from build123d import *

# Parameters (mm, degrees)
BOSS_EXTRUDE1_DEPTH  = 160
SKETCH2_W            = 40
SKETCH2_H            = 2
CUT_EXTRUDE1_DEPTH   = 4
M4_CLEARANCE_HOLE1_D = 4.5
CUT_EXTRUDE2_REACH   = 163.357
SKETCH5_R            = 3.1


with BuildPart() as part:
    # Sketch1 → Boss-Extrude1 (new body)
    with BuildSketch(Plane.XY):
        Polygon((4, -4), (16, -4), (16, -10), (20, -10), (20, 0), (16, 0), (4, 0), align=None)
    extrude(amount=BOSS_EXTRUDE1_DEPTH)

    # Sketch2 → Cut-Extrude1 (cut)
    with BuildSketch(Plane(origin=(20, 0, 0), x_dir=(0, 0, -1), z_dir=(1, 0, 0))):
        with Locations((-140, -9)):
            Rectangle(SKETCH2_W, SKETCH2_H)
    extrude(amount=-CUT_EXTRUDE1_DEPTH, mode=Mode.SUBTRACT)

    # M4 Clearance Hole1 (through all)
    with Locations(Plane(origin=(0, -4, 0), x_dir=(-1, 0, 0), z_dir=(0, -1, 0))):
        with Locations((-10.128911503, -6.267286375), (-10.128911503, -23.38156703), (-10.128911503, -42.093180546), (-10.128911503, -63.314888558), (-9.444340277, -107.583827852), (-9.444340277, -150.244789298)):
            Hole(M4_CLEARANCE_HOLE1_D / 2)

    # Sketch5 → Cut-Extrude2 (cut, up to next)
    with BuildSketch(Plane.XZ.offset(4), mode=Mode.PRIVATE) as cut_extrude2_sk1:
        with Locations(Location((9, 138.897931951, 0), (0, 0, 270))):
            Circle(SKETCH5_R)
    cut_extrude2_tool1 = extrude(cut_extrude2_sk1.sketch, amount=-CUT_EXTRUDE2_REACH, mode=Mode.PRIVATE) & part.part
    add(cut_extrude2_tool1.solids().sort_by_distance((9, -4, 138.897932))[0], mode=Mode.SUBTRACT)


solid = part.part
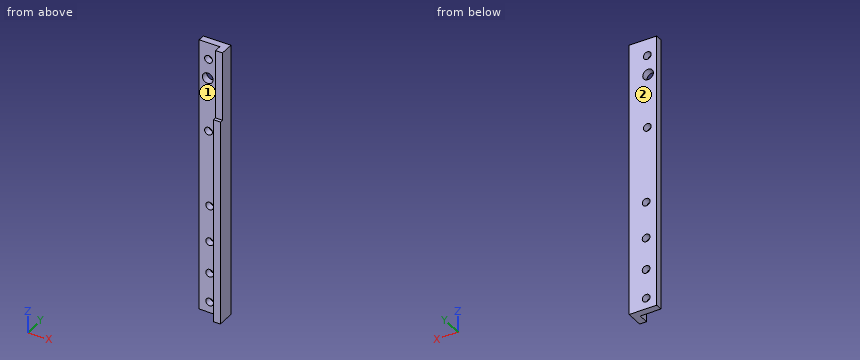
Work out the finished part from the listing and answer in its coordinate system (mm). Face numbers are marked on the shaded views. A direction names the side the tool comes from. Coordinates: 2 decimals unless noted, no trailing zeros. Loops run counter-clockwise (first coordinate to the right, second up) from the corner with the lowest first, then second, coordinate; pieces in that order, holes last. Notation, with made-up numbers: M 44.25,41 L 52.25,41 A24 cw 52.25,66 Z; hole C 49,60.5 d8. An arc over 180 degrees is marked long. Answer in a Markdown table with one row per item. Add a question column.
1. Find section B-B, the plane y = -1.5. Write down the section's boundary in (x, z), then the cut area to 3 significant figures.
2. A tool of negligible diameter and unlimited length cuts with its end or side. For the marked faces 1 and 2, from which of +Z, -Z, +X, -X, +Y, -Y can it reach the whole face along a straight path? Write none if from no direction.
3. Flat-ended cylindrical pins translate along their axes: P1, Ø8, axis at x = 9, z = 138.9, coming from the -Y side; P2, Ø1.6, axis at x = 17.5, y = -9.5, coming from the +Z side; P3, Ø3, axis at y = -6, z = 81.5, coming from the -X side; P4, Ø2.5, axis at x = 10.13, z = 6.27, coming from the -Y side. Find the tip coordinate at first contact, or state that the pin passes through.
4. Find section A-A, the plane z = 69. Write down the section's boundary in (x, y).
5. Consider L1, parallel to X at y = -4.75, z = 126.5; L2, parallel to Y at x = 6.5, z = 106.5; L3, parallel to Z at x = 17, y = -8.25. Determine where each line is inside the solid, lowest interval first.
6. Find section C-C, the plane z = 123. Write down the section's boundary in (x, y).
Reported:
| question | item | result |
|---|---|---|
| 1 | outline | M 4,0 L 20,0 L 20,160 L 4,160 Z; hole C 9,138.9 d6.2; hole C 9.44,107.58 d4.5; hole C 9.44,150.24 d4.5; hole C 10.13,6.27 d4.5; hole C 10.13,23.38 d4.5; hole C 10.13,42.09 d4.5; hole C 10.13,63.31 d4.5 |
| 1 | area | 2,430 mm^2 |
| 2 | face 1 | +Z, -Z, -X, -Y |
| 2 | face 2 | +Z, -Z, +X, -X, +Y |
| 3 | P1 | stops at y = -4 |
| 3 | P2 | stops at z = 120 |
| 3 | P3 | stops at x = 16 |
| 3 | P4 | passes through |
| 4 | outline | M 4,-4 L 16,-4 L 16,-10 L 20,-10 L 20,0 L 4,0 Z |
| 5 | L1 | x = 16 to 20 |
| 5 | L2 | y = -4 to 0 |
| 5 | L3 | z = 0 to 120 |
| 6 | outline | M 4,-4 L 16,-4 L 16,-8 L 20,-8 L 20,0 L 4,0 Z |
